```python
from build123d import *

# Parameters (mm, degrees)
F1_DEPTH  = 40
F3_DEPTH  = 25
F4_DEPTH  = 40
F5_DEPTH  = 14
F6_DEPTH  = 19
F0_W      = 9
F0_H      = 20.0069169636
F7_DEPTH  = 24
F8_DEPTH  = 29
F9_DEPTH  = 34
F10_DEPTH = 10
F0_W_2    = 24.1446838646
F0_H_2    = 9.6578735458
F11_DEPTH = 5
F0_W_3    = 3.2473218008
F0_H_3    = 25.3850887019
F12_DEPTH = 40
F13_DEPTH = 14


with BuildPart() as f1:
    # F0 (on Top) → F1 (new body)
    with BuildSketch(Plane.XY):
        Polygon((-37.1828131515, 17.3178310944), (-37.1828131515, -22.6960028327), (-32.3538763785, -22.6960028327), (-32.3538763785, -13.0381292869), (-32.3538763785, -2.6890858691), (-32.3538763785, 17.3178310944), align=None)
    extrude(amount=F1_DEPTH)

    # F2 (on face) → F3 (cut)
    with BuildSketch(Plane.YZ.offset(-32.3538763785)):
        Polygon((-22.6960028327, 40), (-22.6960028327, 14), (12.3178310944, 40), align=None)
    extrude(amount=-F3_DEPTH, mode=Mode.SUBTRACT)

    # F0 (on Top) → F4 (join)
    with BuildSketch(Plane.XY):
        Polygon((-37.1828131515, 22.6960028327), (-37.1828131515, 17.3178310944), (-32.3538763785, 17.3178310944), (-8.209192514, 17.3178310944), (0.790807486, 17.3178310944), (9.790807486, 17.3178310944), (9.790807486, 22.6960028327), align=None)
    extrude(amount=F4_DEPTH)

    # F0 (on Top) → F5 (join)
    with BuildSketch(Plane.XY):
        Polygon((-8.209192514, -2.6890858691), (-32.3538763785, 17.3178310944), (-32.3538763785, -2.6890858691), align=None)
    extrude(amount=F5_DEPTH)

    # F0 (on Top) → F6 (join)
    with BuildSketch(Plane.XY):
        Polygon((-8.209192514, 17.3178310944), (-32.3538763785, 17.3178310944), (-8.209192514, -2.6890858691), align=None)
    extrude(amount=F6_DEPTH)

    # F0 (on Top) → F7 (join)
    with BuildSketch(Plane.XY):
        with Locations((-3.709192514, 7.3143726126)):
            Rectangle(F0_W, F0_H)
    extrude(amount=F7_DEPTH)

    # F0 (on Top) → F8 (join)
    with BuildSketch(Plane.XY):
        with Locations((5.290807486, 7.3143726126)):
            Rectangle(F0_W, F0_H)
    extrude(amount=F8_DEPTH)

    # F0 (on Top) → F9 (join)
    with BuildSketch(Plane.XY):
        Polygon((33.9354913506, 22.6960028327), (9.790807486, 22.6960028327), (9.790807486, 17.3178310944), (9.790807486, -2.6890858691), (33.9354913506, -2.6890858691), align=None)
    extrude(amount=F9_DEPTH)

    # F0 (on Top) → F10 (join)
    with BuildSketch(Plane.XY):
        Polygon((-32.3538763785, -2.6890858691), (-32.3538763785, -13.0381292869), (-8.209192514, -13.0381292869), (33.9354913506, -13.0381292869), (33.9354913506, -2.6890858691), (9.790807486, -2.6890858691), (0.790807486, -2.6890858691), (-8.209192514, -2.6890858691), align=None)
    extrude(amount=F10_DEPTH)

    # F0 (on Top) → F11 (join)
    with BuildSketch(Plane.XY):
        with Locations((-20.2815344463, -17.8670660598)):
            Rectangle(F0_W_2, F0_H_2)
    extrude(amount=F11_DEPTH)

    # F0 (on Top) → F12 (join)
    with BuildSketch(Plane.XY):
        with Locations((35.559152251, 10.0034584818)):
            Rectangle(F0_W_3, F0_H_3)
    extrude(amount=F12_DEPTH)

    # F0 (on Top) → F13 (join)
    with BuildSketch(Plane.XY):
        Polygon((33.9354913506, -2.6890858691), (33.9354913506, -13.0381292869), (33.9354913506, -22.6960028327), (37.1828131515, -22.6960028327), (37.1828131515, -2.6890858691), align=None)
    extrude(amount=F13_DEPTH)


solid = f1.part
```
The listing builds one solid part. Answer for the finished solid, in the listing's coordinates (mm). A direction names the side the tool comes from. Round coordinates to 2 decimals unless told otherwise and drop trailing zeros. Write each loop counter-clockwise with the first axis right and the second up, starting at its lowest first coordinate (ties: lowest second). Pieces come first, ordered by that corner, then holes. Notation, with made-up numbers: (64, 17.25) -> (118, 17.25) arc R27 cw to (118, 56.25) -> close; hole circle Ø8 at (69.25, -40). An arc over 180 degrees is marked (long way). Use CSV: the item, a comma, the result in double quotes. Start each with the question number.
(1) Section D-D on y = -16.5 is taken. Give the vertices of the cut face in (x, z), then the cut area to 3 significant figures.
(2) Section C-C on z = 36 is taken. Give the vertices of the cut face in (x, y).
(3) The mould has two halves that part along X. Classify faces 5 (the face through (-1, 22.696, 20)), 6 (the face through (-37.183, 5, 15)), 7 (the face through (-12, 17.318, 29)), 8 (the face through (33.935, -15, 8)): released by +X, released by -X, zero draft, split by the parting line, or undercut.
(4) Section B-B on x = -2.5 is taken. Give the vertices of the cut face in (y, z).
(5) Consider L1, parallel to X at y = 1.5, z = 28; L2, parallel to X at y = 15, z = 19.5; L3, parallel to Y at x = 7, z = 16.5. Determine where each line is inside the solid, lowest interval first. Write a range as from..to.
(6) Each of these flat-tipped pins is pushed along its axis until it touches: pin 1 (1 mm diameter, centred on x = 35, y = -11.5, fed in from +Z); pin 2 (6 mm diameter, centred on x = -15, y = 10, fed in from +Z); pin 3 (10 mm diameter, centred on x = 7, y = 9.5, fed in from +Z); pin 4 (10 mm diameter, centred on y = -16, z = 29, fed in from +X). Where does it stop, or does it pass through?
(7) Which of the six approach directions +Z, -Z, +X, -X, +Y, -Y give full straight-line access (tool end or side, diameter ignored) to faces 1 (the face through (9.791, 7, 31)), 2 (the face through (-8.209, -18, 2)), 3 (the face through (36, -13, 14)), 4 (the face through (-34.73, -5.43, 26.82))?
(8) Section A-A on y = 0.5 is taken. Give the vertices of the cut face in (x, z).
A:
1,outline,"(-37.18, 0) -> (-8.21, 0) -> (-8.21, 5) -> (-32.35, 5) -> (-32.35, 18.6) -> (-37.18, 18.6) -> close; (33.94, 0) -> (37.18, 0) -> (37.18, 14) -> (33.94, 14) -> close"
1,area,"256 mm²"
2,outline,"(-37.18, 6.93) -> (-32.35, 6.93) -> (-32.35, 17.32) -> (9.79, 17.32) -> (9.79, 22.7) -> (-37.18, 22.7) -> close; (33.94, -2.69) -> (37.18, -2.69) -> (37.18, 22.7) -> (33.94, 22.7) -> close"
3,face 5,"zero draft"
3,face 6,"released by -X"
3,face 7,"undercut"
3,face 8,"undercut"
4,outline,"(-13.04, 0) -> (22.7, 0) -> (22.7, 40) -> (17.32, 40) -> (17.32, 24) -> (-2.69, 24) -> (-2.69, 10) -> (-13.04, 10) -> close"
5,L1,"x = -37.18..-32.35, 0.79..37.18"
5,L2,"x = -37.18..-32.35, -8.21..37.18"
5,L3,"y = -2.69..22.7"
6,pin 1,"stops at z = 14"
6,pin 2,"stops at z = 19"
6,pin 3,"stops at z = 34"
6,pin 4,"passes through"
7,face 1,"+Z, -Y"
7,face 2,"+Z, -Z, -Y"
7,face 3,"+Z, +X, -Y"
7,face 4,"+Z, -X, -Y"
8,outline,"(-37.18, 0) -> (37.18, 0) -> (37.18, 40) -> (33.94, 40) -> (33.94, 34) -> (9.79, 34) -> (9.79, 29) -> (0.79, 29) -> (0.79, 24) -> (-8.21, 24) -> (-8.21, 19) -> (-12.06, 19) -> (-12.06, 14) -> (-32.35, 14) -> (-32.35, 31.22) -> (-37.18, 31.22) -> close"
